For this review, take the finished solid that the model builds, in its own axes (mm). Coordinates: 2 decimals unless noted, no trailing zeros. Write each loop counter-clockwise with the first axis right and the second up, starting at its lowest first coordinate (ties: lowest second). Pieces come first, ordered by that corner, then holes.
1) Insertion check: P1, Ø5, axis at x = 25, y = -8, coming from the +Z side; P2, Ø2, axis at x = 204.5, y = -14.5, coming from the +Z side; P3, Ø1, axis at y = -18.5, z = 44, coming from the -X side. Each pin has a flat end and moves straight along its axis. Give the tip position at first contact, or say it passes through.
2) We need section A-A on y = -6. Write out the cut boundary in (x, z) (3 decimals), then the cut area to 3 significant figures.
3) We need section C-C on x = 88.5. Write out the cut boundary in (y, z), then the cut area to 3 significant figures.
4) We need section D-D on x = 172. Write out the cut boundary in (y, z).
5) To check wall thickness, follow line 1 along Z through (x, y) = (194, -23); line 2 along Z through (x, y) = (194, -16); line 3 along Z through (x, y) = (203, -19.05) (3 decimals). State the ranges of each line that lie inside material, in increasing order.
from build123d import *

# Parameters (mm, degrees)
F1_DEPTH = 38.1
F2_R     = 5.08
F3_DEPTH = 38.1
F4_R     = 9.525
F5_DEPTH = 53.34
F6_R     = 1.905
F7_DEPTH = 38.101
F8_DEPTH = 38.101


# Not quite as in the source:
# - a feature names something its author has since deleted; it is built from what else it names


with BuildPart() as f1:
    # F0 (on Front) → F1 (new body)
    with BuildSketch(Plane.XZ):
        with BuildLine():
            ThreePointArc((140.9522952768, 27.729119938), (69.5233725404, 18.7076937305), (0, 0))
            Line((0, 0), (228.6, 0))
            Line((228.6, 0), (228.6, 25.4))
            ThreePointArc((228.6, 25.4), (184.8248483375, 28.3972283618), (140.9522952768, 27.729119938))
        make_face()
    extrude(amount=F1_DEPTH)

    # F2
    f2_edges = [f1.edges().sort_by_distance(p)[0] for p in [
        (112.892107, 0, 25.371039),
        (112.892107, -38.1, 25.371039),
    ]]
    fillet(f2_edges, radius=F2_R)

    # F0 (on Front) → F3 (join)
    with BuildSketch(Plane.XZ):
        with BuildLine():
            ThreePointArc((140.9522952768, 27.729119938), (69.5233725404, 18.7076937305), (0, 0))
            Line((0, 0), (228.6, 0))
            Line((228.6, 0), (228.6, 25.4))
            ThreePointArc((228.6, 25.4), (184.8248483375, 28.3972283618), (140.9522952768, 27.729119938))
        make_face()
        with BuildLine():
            ThreePointArc((228.6, 69.85), (187.9185150392, 42.2507295914), (140.9522952768, 27.729119938))
            ThreePointArc((140.9522952768, 27.729119938), (184.8248483375, 28.3972283618), (228.6, 25.4))
            Line((228.6, 25.4), (228.6, 69.85))
        make_face()
    extrude(amount=F3_DEPTH)

    # F4 (on face) → F5 (cut)
    with BuildSketch(Plane.YZ.offset(228.6)):
        with Locations((-19.05, 25.4)):
            Circle(F4_R)
    extrude(amount=-F5_DEPTH, mode=Mode.SUBTRACT)

    # F6 (on face) → F7 (cut, through all)
    with BuildSketch(Plane.XZ.offset(38.1)):
        with Locations((76.2, 3.81)):
            Circle(F6_R)
    extrude(amount=-F7_DEPTH, mode=Mode.SUBTRACT)

    # F6 (on face) → F8 (cut, through all)
    with BuildSketch(Plane.XZ.offset(38.1)):
        with Locations((194.31, 3.81)):
            Circle(F6_R)
    extrude(amount=-F8_DEPTH, mode=Mode.SUBTRACT)


solid = f1.part
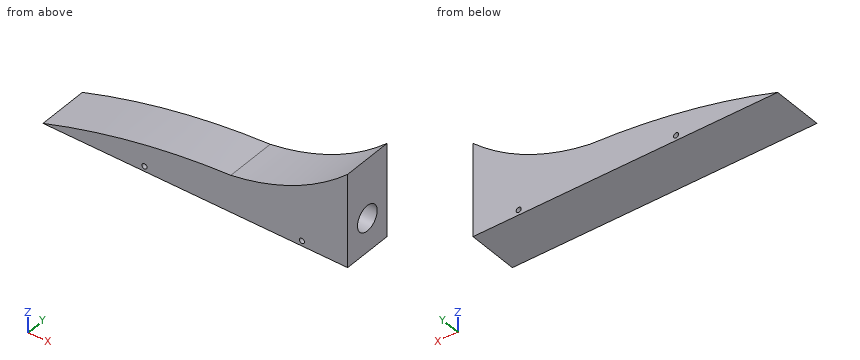
Result:
1. P1: stops at z = 8.63
1. P2: stops at z = 52.05
1. P3: stops at x = 190.46
2. outline: (0, 0) - (228.6, 0) - (228.6, 69.85) arc R166.561 cw to (140.952, 27.729) arc R525.073 ccw to start; hole circle Ø3.81 at (76.2, 3.81); hole circle Ø3.81 at (194.31, 3.81)
2. area: 6,210 mm2
3. outline: (-38.1, 0) - (0, 0) - (0, 22.08) - (-38.1, 22.08) - close
3. area: 841 mm2
4. outline: (-38.1, 0) - (0, 0) - (0, 35.59) - (-38.1, 35.59) - close
5. line 1: z = 0 to 1.93, 5.69 to 16.73, 34.07 to 45.33
5. line 2: z = 0 to 1.93, 5.69 to 16.38, 34.42 to 45.33
5. line 3: z = 0 to 15.875, 34.925 to 50.482
